Autodesk Inventor part; units mm, degrees
ref_plane "YZ Plane" through (0, 0, 0) normal (1, 0, 0) x (0, 1, 0)
ref_plane "XZ Plane" through (0, 0, 0) normal (0, 1, 0) x (-1, 0, 0)
ref_plane "XY Plane" through (0, 0, 0) normal (0, 0, 1) x (1, 0, 0)
sketch "Sketch_1" plane through (0, 0, 0) normal (1, 0, 0) x (0, 1, 0)
  line L0 (50.8, 22.225) -> (10.16, 22.225)
  arc A0 (10.16, 22.225) -> (0, 12.065) centre (10.16, 12.065) ccw
  line L1 (0, 12.065) -> (0, -12.065)
  arc A1 (0, -12.065) -> (10.16, -22.225) centre (10.16, -12.065) ccw
  line L2 (10.16, -22.225) -> (50.8, -22.225)
  line L3 (50.8, -22.225) -> (50.8, 22.225)
extrude "Extrusion1" add sketch "Sketch_1" along normal mid plane 132.1816
sketch "Sketch_10" plane through (0, 0, 0) normal (0, 1, 0) x (-1, 0, 0)
  circle A0 centre (0, 0) radius 132.1816
  arc A1 (43.8658, -22.225) -> (43.8658, 22.225) centre (43.8658, 0) ccw
  line L0 (43.8658, 22.225) -> (-43.8658, 22.225)
  arc A2 (-43.8658, 22.225) -> (-43.8658, -22.225) centre (-43.8658, 0) ccw
  line L1 (-43.8658, -22.225) -> (43.8658, -22.225)
extrude "Extrusion2" cut sketch "Sketch_10" along normal blind 50.8
sketch "Sketch_7" plane through (0, 0, 0) normal (0, 0, 1) x (1, 0, 0)
  line L0 (86.8172, 25.4) -> (10.3632, 25.4)
  line L1 (10.3632, 25.4) -> (10.3632, 46.1433)
  arc A0 (11.8449, 47.625) -> (10.3632, 46.1433) centre (11.8449, 46.1433) ccw
  line L2 (11.8449, 47.625) -> (85.3355, 47.625)
  arc A1 (86.8172, 46.1433) -> (85.3355, 47.625) centre (85.3355, 46.1433) ccw
  line L3 (86.8172, 46.1433) -> (86.8172, 25.4)
  line L4 (86.8172, 25.4) -> (10.3632, 25.4)
revolve "Revolution1" add sketch "Sketch_7" angle 360 about axis through (86.8172, 25.4, 0) along (1, 0, 0)
sketch "Sketch_14" plane through (-43.8658, 0, 0) normal (1, 0, 0) x (0, 0, -1)
  line L0 (42.8498, 25.4) -> (0, 25.4)
  line L1 (0, 25.4) -> (0, 47.625)
  line L2 (0, 47.625) -> (41.3681, 47.625)
  arc A0 (42.8498, 46.1433) -> (41.3681, 47.625) centre (41.3681, 46.1433) ccw
  line L3 (42.8498, 46.1433) -> (42.8498, 25.4)
  line L4 (42.8498, 25.4) -> (0, 25.4)
revolve "Revolution2" add sketch "Sketch_14" angle 360 about axis through (-43.8658, 25.4, -42.8498) along (0, 0, -1)
sketch "Sketch_15" plane through (0, 0, 0) normal (1, 0, 0) x (0, 1, 0)
  line L0 (50.8, 17.145) -> (0, 17.145)
  arc A0 (0, 17.145) -> (-7.62, 9.525) centre (0, 9.525) ccw
  line L1 (-7.62, 9.525) -> (-7.62, -9.525)
  arc A1 (-7.62, -9.525) -> (0, -17.145) centre (0, -9.525) ccw
  line L2 (0, -17.145) -> (50.8, -17.145)
  line L3 (50.8, -17.145) -> (50.8, 17.145)
sketch "Sketch_17" plane through (0, 0, 0) normal (0, 0, 1) x (1, 0, 0)
  line L0 (-43.8912, -7.62) -> (-43.8912, 50.8)
  line L1 (-43.8912, 50.8) -> (-26.7462, 50.8)
  line L2 (-26.7462, 50.8) -> (-26.7462, 0)
  arc A0 (-34.3662, -7.62) -> (-26.7462, 0) centre (-34.3662, 0) ccw
  line L3 (-34.3662, -7.62) -> (-43.8912, -7.62)
  line L4 (-43.8912, -7.62) -> (-43.8912, 50.8)
revolve "Revolution3" cut sketch "Sketch_17" angle 360 about axis through (-43.8912, -7.62, 0) along (0, -1, 0)
extrude "Extrusion3" cut sketch "Sketch_15" along normal mid plane 87.7824
sketch "Sketch_3" plane through (0, 0, 0) normal (0, 0, 1) x (1, 0, 0)
  line L0 (43.8912, -7.62) -> (43.8912, 50.8)
  line L1 (43.8912, 50.8) -> (61.0362, 50.8)
  line L2 (61.0362, 50.8) -> (61.0362, 0)
  arc A0 (53.4162, -7.62) -> (61.0362, 0) centre (53.4162, 0) ccw
  line L3 (53.4162, -7.62) -> (43.8912, -7.62)
  line L4 (43.8912, -7.62) -> (43.8912, 50.8)
revolve "Revolution4" cut sketch "Sketch_3" angle 360 about axis through (43.8912, -7.62, 0) along (0, -1, 0)
sketch "Sketch_8" plane through (0, 50.8, 0) normal (0, 1, 0) x (1, 0, 0)
  arc A0 (57.785, -13.9449) -> (57.785, 13.9449) centre (43.8912, 0) ccw
  line L0 (57.785, 13.9449) -> (57.785, -13.9449)
extrude "Extrusion4" add sketch "Sketch_8" against normal blind 2.54
sketch "Sketch_9" plane through (0, 50.8, 0) normal (0, 1, 0) x (1, 0, 0)
  arc A0 (-57.785, 13.9449) -> (-57.785, -13.9449) centre (-43.8912, 0) ccw
  line L0 (-57.785, -13.9449) -> (-57.785, 13.9449)
extrude "Extrusion5" add sketch "Sketch_9" against normal blind 2.54
sketch "Sketch_4" plane through (0, 0, 0) normal (0, 1, 0) x (-1, 0, 0)
  arc A0 (-57.785, 13.9449) -> (-57.785, -13.9449) centre (-43.8912, 0) ccw
  line L0 (-57.785, -13.9449) -> (-57.785, 13.9449)
extrude "Extrusion6" add sketch "Sketch_4" along normal blind 2.54
sketch "Sketch_5" plane through (0, 0, 0) normal (0, 1, 0) x (-1, 0, 0)
  arc A0 (57.785, -13.9449) -> (57.785, 13.9449) centre (43.8912, 0) ccw
  line L0 (57.785, 13.9449) -> (57.785, -13.9449)
extrude "Extrusion7" add sketch "Sketch_5" along normal blind 2.54
sketch "Sketch_6" plane through (0, 0, 0) normal (1, 0, 0) x (0, 1, 0)
  line L0 (2.54, 22.225) -> (-50.8, 22.225)
  line L1 (-50.8, 22.225) -> (-50.8, -22.225)
  line L2 (-50.8, -22.225) -> (2.54, -22.225)
  line L3 (2.54, -22.225) -> (2.54, -18.7852)
  arc A0 (0, -12.065) -> (2.54, -18.7852) centre (10.16, -12.065) ccw
  line L4 (0, -12.065) -> (0, 12.065)
  arc A1 (2.54, 18.7852) -> (0, 12.065) centre (10.16, 12.065) ccw
  line L5 (2.54, 18.7852) -> (2.54, 22.225)
extrude "Extrusion8" cut sketch "Sketch_6" along normal mid plane 132.1816
sketch "Sketch_11" plane through (0, 0, 0) normal (0, 0, 1) x (1, 0, 0)
  line L0 (86.8172, 25.4) -> (10.3632, 25.4)
  line L1 (10.3632, 25.4) -> (10.3632, 38.9999)
  line L2 (10.3632, 38.9999) -> (85.3511, 41.341)
  line L3 (85.3511, 41.341) -> (86.8172, 42.8536)
  line L4 (86.8172, 42.8536) -> (86.8172, 25.4)
  line L5 (86.8172, 25.4) -> (10.3632, 25.4)
revolve "Revolution5" cut sketch "Sketch_11" angle 360 about axis through (86.8172, 25.4, 0) along (1, 0, 0)
thread "Thread1"
sketch "Sketch_12" plane through (-43.8658, 0, 0) normal (1, 0, 0) x (0, 0, -1)
  line L0 (42.8498, 25.4) -> (0, 25.4)
  line L1 (0, 25.4) -> (0, 40.049)
  line L2 (0, 40.049) -> (41.3837, 41.341)
  line L3 (41.3837, 41.341) -> (42.8498, 42.8536)
  line L4 (42.8498, 42.8536) -> (42.8498, 25.4)
  line L5 (42.8498, 25.4) -> (0, 25.4)
revolve "Revolution6" cut sketch "Sketch_12" angle 360 about axis through (-43.8658, 25.4, -42.8498) along (0, 0, -1)
thread "Thread2"
properties part number "L37-TB"
Can you work these out from the model? Positions are in its coordinate system, mm. A direction names the side the tool comes from. Give positions to 0.01 mm unless a question says otherwise; leave off trailing zeros. Loops run counter-clockwise (first coordinate to the right, second up) from the corner with the lowest first, then second, coordinate; pieces in that order, holes last. Notation, with made-up numbers: (49.5, 78) - (100.5, 78) arc R13 cw to (100.5, 99) - close; hole circle Ø4 at (53.25, 28.25). An arc over 180 degrees is marked (long way). One line per item, written item: value.
(1) If we section it at D-D, the plane z = -32.5: List the corners of the cut face in (x, y) for me (3 decimals).
Verdict:
outline: circle Ø44.45 at (-43.866, 25.4); hole circle Ø31.327 at (-43.866, 25.4)
(2) If we section it at B-B, the plane z = 5: State how many separate pieces and enclosed holes the cut face has, plus the area to 3 significant figures.
Verdict:
separate pieces: 3
enclosed holes: 0
area: 694 mm^2
(3) If we section it at A-A, the plane x = -19.5: List the corners of the cut face in (y, z) for me (3 decimals).
Verdict:
outline: (1.361, -17.145) arc R10.16 ccw to (10.16, -22.225) - (50.8, -22.225) - (50.8, -17.145) - close; (1.361, 17.145) - (50.8, 17.145) - (50.8, 22.225) - (10.16, 22.225) arc R10.16 ccw to start
(4) If we mould it in two halves opening along Y, with no side actions, what happens to faces 4 (the face through (59, 48.26, 0)), 5 (the face through (69.082, 14.025, 10.43)), 6 (the face through (-5, 50.8, -18)), 7 (the face through (-1, 31, 22.225))? For each: released by +Y, released by -Y, zero draft, split by the parting line, or undercut.
Verdict:
face 4: undercut
face 5: undercut
face 6: released by +Y
face 7: zero draft
(5) I need wall thicknesses on line 1 along X through (y, z) = (8, 1); line 2 along Z through (x, y) = (38, 38.5) (3 decimals); line 3 along X through (y, z) = (44.5, 4.5). Which ranges of each line are inside material? Lowest first, please.
Verdict:
line 1: -66.07 to -61.01, 61.01 to 86.79
line 2: -22.225 to -17.145, 17.145 to 22.225
line 3: -65.63 to -60.44, 60.44 to 86.82
(6) On a 3-axis mill with a long thin cutter (end or side, diameter ignored), from which of +Z, -Z, +X, -X, +Y, -Y can I reach the whole of each face in a straight line? I mean faces 1 (the face through (-65.56, 20.58, -30.17)), 2 (the face through (-59, 48.26, 0)), 3 (the face through (-59, 16, -42.85)). Say none if no direction works.
Verdict:
face 1: -Z
face 2: none
face 3: -Z, +X, -X, +Y, -Y
(7) I'm going to push flat-ended pins straight in: pin 1 (3.5 mm diameter, centred on x = 59, z = 4, fed in from -Y); pin 2 (5 mm diameter, centred on y = 28.5, z = -31.5, fed in from +X); pin 3 (3 mm diameter, centred on y = 1, z = -0.5, fed in from +X); pin 4 (4 mm diameter, centred on y = 10, z = -29.5, fed in from +X). Where does each tip first touch, or does it pass through?
Verdict:
pin 1: y = 0
pin 2: x = -21.65
pin 3: x = 66.09
pin 4: x = -26.13
